Check sheet for the modelled part. Datum: model origin and axes. Units: mm. A direction names the side the tool comes from. Give positions to 0.01 mm unless a question says otherwise; leave off trailing zeros. Answer in a Markdown table with one row per item.
from build123d import *

# Parameters (mm, degrees)
SKETCH1_R           = 2
BOSS_EXTRUDE1_DEPTH = 119
FILLET1_R           = 1
FILLET2_R           = 0.5
FILLET4_R           = 0.5


with BuildPart() as part:
    # Sketch1 → Boss-Extrude1 (new body)
    with BuildSketch(Plane(origin=(0, 0, 0), x_dir=(1, 0, 0), z_dir=(0, 1, 0))):
        Polygon((7, 18), (7, 20), (0, 20), (0, 13), (2, 13), (2, 17), (6, 13), (6, 10.5), (6.5, 10), (6, 9.5), (6, 7), (2, 3), (2, 7), (0, 7), (0, 0), (7, 0), (7, 2), (3, 2), (7, 6), (9.5, 6), (10, 6.5), (10.5, 6), (13, 6), (17, 2), (13, 2), (13, 0), (20, 0), (20, 7), (18, 7), (18, 3), (14, 7), (14, 9.5), (13.5, 10), (14, 10.5), (14, 13), (18, 17), (18, 13), (20, 13), (20, 20), (13, 20), (13, 18), (17, 18), (13, 14), (10.5, 14), (10, 13.5), (9.5, 14), (7, 14), (3, 18), align=None)
        with Locations((10, 10)):
            Circle(SKETCH1_R, mode=Mode.SUBTRACT)
    extrude(amount=BOSS_EXTRUDE1_DEPTH)

    # Fillet1
    fillet1_edges = [part.edges().sort_by_distance(p)[0] for p in [
        (20, 59.5, 0),
        (0, 59.5, 0),
        (0, 59.5, -20),
        (20, 59.5, -20),
    ]]
    fillet(fillet1_edges, radius=FILLET1_R)

    # Fillet2
    fillet2_edges = [part.edges().sort_by_distance(p)[0] for p in [
        (18, 59.5, -7),
        (20, 59.5, -7),
        (13, 59.5, 0),
        (13, 59.5, -2),
        (7, 59.5, -2),
        (7, 59.5, 0),
        (0, 59.5, -7),
        (2, 59.5, -7),
        (2, 59.5, -13),
        (0, 59.5, -13),
        (7, 59.5, -20),
        (7, 59.5, -18),
        (13, 59.5, -18),
        (13, 59.5, -20),
        (20, 59.5, -13),
        (18, 59.5, -13),
    ]]
    fillet(fillet2_edges, radius=FILLET2_R)

    # Fillet4
    fillet4_edges = [part.edges().sort_by_distance(p)[0] for p in [
        (10.5, 59.5, -6),
        (9.5, 59.5, -6),
        (6, 59.5, -9.5),
        (6, 59.5, -10.5),
        (9.5, 59.5, -14),
        (10.5, 59.5, -14),
        (14, 59.5, -10.5),
        (14, 59.5, -9.5),
    ]]
    fillet(fillet4_edges, radius=FILLET4_R)


solid = part.part
(1) Access from +Z, -Z, +X, -X, +Y, -Y to the whole of each face (thin tool, end or side, straight path). Record for faces 1 (the flat face through (6, 59, -12)), 2 (the flat face through (14, 59, -8)), 3 (the flat face through (8, 59, -6)), 4 (the flat face through (16, 59, 0)).
Geometry says:
| item | result |
|---|---|
| face 1 | -X, +Y, -Y |
| face 2 | +X, +Y, -Y |
| face 3 | +Z, +Y, -Y |
| face 4 | +Z, +X, -X, +Y, -Y |
(2) Mould release check, pull along Z, two halves, no side actions. Record for faces 5 (the flat face through (8, 59, -14)), 6 (the flat face through (0, 59, -4)), 7 (the flat face through (15, 59, -4)), 8 (the flat face through (4, 59, 0)): pulls with the +Z half, pulls with the -Z half, needs draft (parallel to the pull), parting line crosses it, or undercut.
Geometry says:
| item | result |
|---|---|
| face 5 | pulls with the -Z half |
| face 6 | needs draft |
| face 7 | undercut |
| face 8 | pulls with the +Z half |
(3) Thickness scan on L1, parallel to Z at x = 10, y = 28; L2, parallel to X at y = 27, z = -10; L3, parallel to X at y = 14.5, z = -4.25. Record the ranges inside material, lowest first.
Geometry says:
| item | result |
|---|---|
| L1 | -13.5 to -12, -8 to -6.5 |
| L2 | 6.5 to 8, 12 to 13.5 |
| L3 | 0 to 2, 3.25 to 5.25, 14.75 to 16.75, 18 to 20 |
(4) Gauge pin test, flat ends, axial feed: P1, Ø1.1, axis at y = 62, z = -12, coming from the -X side; P2, Ø0.7, axis at x = 12, y = 53, coming from the -Z side; P3, Ø12, axis at y = 106, z = -8.5, coming from the -X side; P4, Ø1.5, axis at x = 9, y = 16.5, coming from the +Z side. Record the tip position at first contact, or that the pin passes through.
Geometry says:
| item | result |
|---|---|
| P1 | x = 6 |
| P2 | z = -14 |
| P3 | x = 0 |
| P4 | z = -6 |
